```python
from build123d import *

# Parameters (mm, degrees)
SKETCH1_W           = 72
SKETCH1_H           = 72
BOSS_EXTRUDE1_DEPTH = 400
RIB2_START          = -3
RIB2_DEPTH          = 6
BOSS_EXTRUDE2_DEPTH = 3


# Read off the part's stored shape, not the designer's step: Rib2
with BuildPart() as part:
    # Sketch1 → Boss-Extrude1 (new body)
    with BuildSketch(Plane(origin=(0, 0, 0), x_dir=(1, 0, 0), z_dir=(0, 1, 0))):
        with BuildLine():
            Line((2, 0), (78, 0))
            ThreePointArc((78, 0), (79.414213562, 0.585786438), (80, 2))
            Line((80, 2), (80, 78))
            ThreePointArc((80, 78), (79.414213562, 79.414213562), (78, 80))
            Line((78, 80), (2, 80))
            ThreePointArc((2, 80), (0.585786438, 79.414213562), (0, 78))
            Line((0, 78), (0, 2))
            ThreePointArc((0, 2), (0.585786438, 0.585786438), (2, 0))
        make_face()
        with Locations((40, 40)):
            Rectangle(SKETCH1_W, SKETCH1_H, mode=Mode.SUBTRACT)
    extrude(amount=BOSS_EXTRUDE1_DEPTH)

    # Rib2 outline → Rib2 (add)
    with BuildSketch(Plane.ZY.offset(-40).offset(RIB2_START)):
        Polygon((0, 80), (0, 0), (30, 0), align=None)
    rib2 = extrude(amount=RIB2_DEPTH)

    # Mirror1: Rib2 across plane
    add(rib2.mirror(Plane(origin=(0, 0, -40), x_dir=(1, 0, 0), z_dir=(0, 0, -1))))

    # Sketch4 → Boss-Extrude2 (add, symmetric)
    with BuildSketch(Plane(origin=(0, 0, -40), x_dir=(-1, 0, 0), z_dir=(0, 0, -1))):
        Polygon((50, 0), (0, 120), (0, 0), align=None)
    extrude(amount=BOSS_EXTRUDE2_DEPTH, both=True)


solid = part.part
```
Geometry check sheet. Reference: the model listing, model coordinates, mm. A direction names the side the tool comes from. Give positions to 0.01 mm unless a question says otherwise; leave off trailing zeros. Loops run counter-clockwise (first coordinate to the right, second up) from the corner with the lowest first, then second, coordinate; pieces in that order, holes last. Notation, with made-up numbers: (-31, 46) - (-3, 46) arc R8 ccw to (-3, 61) - close; hole circle Ø3 at (9, 61.5). An arc over 180 degrees is marked (long way). Use CSV: the item, a comma, the result in double quotes. Start each with the question number.
Q1. Go/stop test with flat-tipped pins: pin 1 Ø24 at (y, z) = (46.5, -89) entering from -X; pin 2 Ø15 at (x, y) = (-36.5, 37) entering from -Z; pin 3 Ø3 at (x, y) = (27, 237.5) entering from +Z. Record where each tip stops, or that it passes through.
Q2. Access from +Z, -Z, +X, -X, +Y, -Y to the whole of each face (thin tool, end or side, straight path). Record for faces 1 (the face through (76, 197, -39)), 2 (the face through (-14, 34, -43)), 3 (the face through (-25.35, 59.16, -40.04)), 4 (the face through (43, 23, -88)).
Q3. Section check C-C, the plane y = 304.5. Record the cut outline in (x, z).
Q4. Section check A-A, the plane z = -49. Record the cut outline in (x, y).
Q5. Scan lines: probe 1 along X at (y, z) = (186, -16); probe 2 along Z at (x, y) = (19.5, 200.5); probe 3 along Z at (x, y) = (-3, 80). Record each from-to range of solid material in increasing order. Write a range as from..to.
Q6. Release check for a two-part mould opening along X. For faces 5 (the face through (4, 197, -39)), 6 (the face through (37, 23, 8)), 7 (the face through (-14, 34, -37)), 8 (the face through (43, 23, 8)) record: +X half, -X half, draft (parallel to the pull), parting line (faces both ways), or undercut.
Q7. Section check B-B, the plane x = 13. Record the cut outline in (y, z).
Q8. Section check D-D, the plane y = 96. Record the cut outline in (x, z).
Findings below:
1,pin 1,"stops at x = 0"
1,pin 2,"stops at z = -43"
1,pin 3,"stops at z = 0"
2,face 1,"+Y, -Y"
2,face 2,"-Z, -X, +Y, -Y"
2,face 3,"+Z, -Z, -X, +Y"
2,face 4,"-Z, +X, +Y, -Y"
3,outline,"(0, -78) arc R2 ccw to (2, -80) - (78, -80) arc R2 ccw to (80, -78) - (80, -2) arc R2 ccw to (78, 0) - (2, 0) arc R2 ccw to (0, -2) - close; hole (4, -76) - (76, -76) - (76, -4) - (4, -4) - close"
4,outline,"(0, 0) - (4, 0) - (4, 400) - (0, 400) - close; (76, 0) - (80, 0) - (80, 400) - (76, 400) - close"
5,probe 1,"x = 0..4, 76..80"
5,probe 2,"z = -80..-76, -4..0"
5,probe 3,"z = -43..-37"
6,face 5,"undercut"
6,face 6,"-X half"
6,face 7,"draft"
6,face 8,"+X half"
7,outline,"(0, -80) - (400, -80) - (400, -76) - (0, -76) - close; (0, -4) - (400, -4) - (400, 0) - (0, 0) - close"
8,outline,"(-10, -43) - (0, -43) - (0, -78) arc R2 ccw to (2, -80) - (78, -80) arc R2 ccw to (80, -78) - (80, -2) arc R2 ccw to (78, 0) - (2, 0) arc R2 ccw to (0, -2) - (0, -37) - (-10, -37) - close; hole (4, -76) - (76, -76) - (76, -4) - (4, -4) - close"
